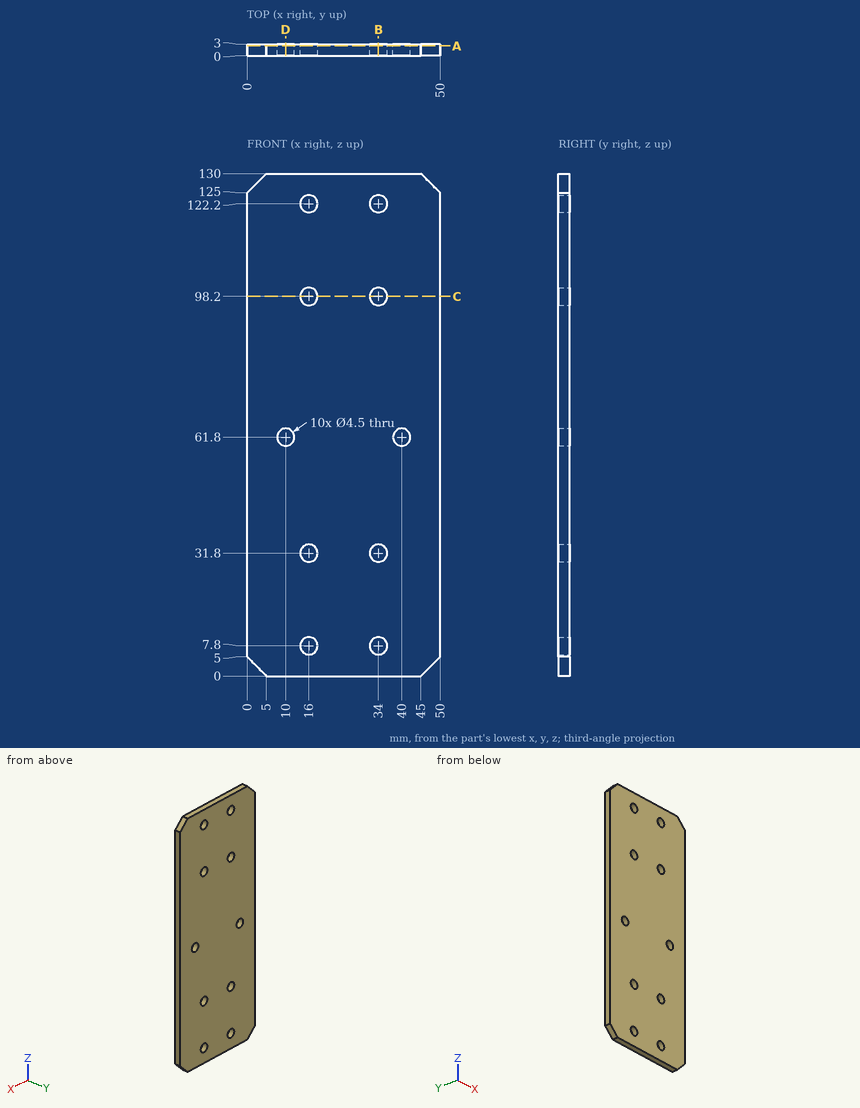
The drawing under review shows one solid part. Ordinate dimensions are in mm from its lowest x, y, z. Coordinates: 2 decimals unless noted, no trailing zeros. Write each loop counter-clockwise with the first axis right and the second up, starting at its lowest first coordinate (ties: lowest second). Pieces come first, ordered by that corner, then holes.
1) Add section B-B (x = 34). Write out the cut boundary in (y, z), plus the area to 3 significant figures.
2) Add section A-A (y = 2.5). State how many separate pieces and enclosed holes the cut face has, plus the area to 3 significant figures.
3) Add section D-D (x = 10). Write out the cut boundary in (y, z).
4) Insertion check: pin 1 (2.5 mm diameter, centred on x = 16, z = 31.8, fed in from -Y). The pin has a flat end and moves straight along its axis. Give the tip position at first contact, or say it passes through.
5) To check wall thickness, follow L1, parallel to Z at x = 16, y = 0.75; L2, parallel to Z at x = 17, y = 0.65; L3, parallel to X at y = 2.6, z = 61.5. State the ranges of each line that lie inside material, in increasing order.
6) Add section C-C (z = 98.2). Write out the cut boundary in (x, y).
Check result:
1. outline: (0, 0) - (3, 0) - (3, 5.55) - (0, 5.55) - close; (0, 10.05) - (3, 10.05) - (3, 29.55) - (0, 29.55) - close; (0, 34.05) - (3, 34.05) - (3, 95.95) - (0, 95.95) - close; (0, 100.45) - (3, 100.45) - (3, 119.95) - (0, 119.95) - close; (0, 124.45) - (3, 124.45) - (3, 130) - (0, 130) - close
1. area: 336 mm2
2. separate pieces: 1
2. enclosed holes: 10
2. area: 6,290 mm2
3. outline: (0, 0) - (3, 0) - (3, 59.55) - (0, 59.55) - close; (0, 64.05) - (3, 64.05) - (3, 130) - (0, 130) - close
4. pin 1: passes through
5. L1: z = 0 to 5.55, 10.05 to 29.55, 34.05 to 95.95, 100.45 to 119.95, 124.45 to 130
5. L2: z = 0 to 5.78, 9.82 to 29.78, 33.82 to 96.18, 100.22 to 120.18, 124.22 to 130
5. L3: x = 0 to 7.77, 12.23 to 37.77, 42.23 to 50
6. outline: (0, 0) - (13.75, 0) - (13.75, 3) - (0, 3) - close; (18.25, 0) - (31.75, 0) - (31.75, 3) - (18.25, 3) - close; (36.25, 0) - (50, 0) - (50, 3) - (36.25, 3) - close
